The listing builds one solid part. Answer for the finished solid, in the listing's coordinates (mm). Face numbers are marked on the shaded views. A direction names the side the tool comes from. Give positions to 0.01 mm unless a question says otherwise; leave off trailing zeros. Order: outer loops, then holes, each group sorted by start corner. A loop starts at its lowest first (then second) coordinate and runs counter-clockwise, first axis right, second up. Notation, with made-up numbers: M -15,-14 L 29,-14 A24 ccw 29,-3 Z; hole C 70.25,64 d9. An arc over 180 degrees is marked long. Answer as a JSON object with one key per item and string values. Group by question number.
```python
from build123d import *

# Parameters (mm, degrees)
F0_W        = 63.5
F0_H        = 50.8
F1_DEPTH    = 3.175
F2_R        = 22.621875
F3_DEPTH    = 1.27
F5_DEPTH    = 25.4
F7_DEPTH    = 50.8
F8_T1_DEPTH = 50.8
F8_T3_DEPTH = 74.3464301965
F8_T5_DEPTH = 76.2
F9_R        = 5.08
F10_R       = 1.27


# Not quite as in the source:
# - a fillet or chamfer that OpenCascade refuses, or shapes differently, is made with other operations: its cross-section is extruded or revolved along the edge and cut away or added


with BuildPart() as f1:
    # F0 (on Right) → F1 (new body)
    with BuildSketch(Plane.YZ):
        Rectangle(F0_W, F0_H)
    extrude(amount=F1_DEPTH)

    # F2 (on face) → F3 (cut)
    with BuildSketch(Plane.YZ.offset(3.175)):
        with Locations((2.778125, 0)):
            Circle(F2_R)
    extrude(amount=-F3_DEPTH, mode=Mode.SUBTRACT)

    # F4 (on face) → F5 (cut)
    with BuildSketch(Plane.YZ.offset(1.905)):
        with BuildLine():
            ThreePointArc((14.3248105234, 15.875), (11.3272476722, 18.1751108739), (9.8813375306, 14.684375))
            Line((9.8813375306, 14.684375), (11.9435605234, 15.875))
            Line((11.9435605234, 15.875), (11.9435605234, 13.49375))
            ThreePointArc((11.9435605234, 13.49375), (13.6273585461, 14.1912019773), (14.3248105234, 15.875))
        make_face()
        with BuildLine():
            Line((-15.5527460468, 0), (-13.490523054, 1.190625))
            ThreePointArc((-13.490523054, 1.190625), (-17.9339960468, 0), (-13.490523054, -1.190625))
            Line((-13.490523054, -1.190625), (-15.5527460468, 0))
        make_face()
        with BuildLine():
            ThreePointArc((-13.490523054, -1.190625), (-13.2526351729, -0.6163128512), (-13.1714960468, 0))
            Line((-13.1714960468, 0), (-15.5527460468, 0))
            Line((-15.5527460468, 0), (-13.490523054, -1.190625))
        make_face()
        with BuildLine():
            Line((-15.5527460468, 0), (-13.1714960468, 0))
            ThreePointArc((-13.1714960468, 0), (-13.2526351729, 0.6163128512), (-13.490523054, 1.190625))
            Line((-13.490523054, 1.190625), (-15.5527460468, 0))
        make_face()
        with BuildLine():
            ThreePointArc((10.7529355234, -13.8127770072), (10.2597625007, -14.1912019773), (9.8813375306, -14.684375))
            Line((9.8813375306, -14.684375), (11.9435605234, -15.875))
            Line((11.9435605234, -15.875), (10.7529355234, -13.8127770072))
        make_face()
        with BuildLine():
            Line((11.9435605234, 15.875), (10.7529355234, 13.8127770072))
            ThreePointArc((10.7529355234, 13.8127770072), (11.3272476722, 13.5748891261), (11.9435605234, 13.49375))
            Line((11.9435605234, 13.49375), (11.9435605234, 15.875))
        make_face()
        with BuildLine():
            Line((11.9435605234, 15.875), (9.8813375306, 14.684375))
            ThreePointArc((9.8813375306, 14.684375), (10.2597625007, 14.1912019773), (10.7529355234, 13.8127770072))
            Line((10.7529355234, 13.8127770072), (11.9435605234, 15.875))
        make_face()
        with BuildLine():
            Line((11.9435605234, -15.875), (9.8813375306, -14.684375))
            ThreePointArc((9.8813375306, -14.684375), (11.3272476722, -18.1751108739), (14.3248105234, -15.875))
            ThreePointArc((14.3248105234, -15.875), (13.6273585461, -14.1912019773), (11.9435605234, -13.49375))
            Line((11.9435605234, -13.49375), (11.9435605234, -15.875))
        make_face()
        with BuildLine():
            ThreePointArc((11.9435605234, -13.49375), (11.3272476722, -13.5748891261), (10.7529355234, -13.8127770072))
            Line((10.7529355234, -13.8127770072), (11.9435605234, -15.875))
            Line((11.9435605234, -15.875), (11.9435605234, -13.49375))
        make_face()
    extrude(amount=-F5_DEPTH, mode=Mode.SUBTRACT)

    # F6 (on face) → F7 (join, through all)
    with BuildSketch(Plane.XY.offset(25.4)):
        Polygon((-19.05, -31.75), (0, -31.75), (0, -28.575), (-15.875, -28.575), (-15.875, -22.225), (-19.05, -22.225), align=None)
    extrude(amount=-F7_DEPTH)

    # F8: fillet of radius 5.08 on 3 edges, made by hand

    # F8_s2 → F8_t1 (join)
    with BuildSketch(Plane.XY.offset(-25.4)):
        with BuildLine():
            ThreePointArc((-5.08, -28.575), (-1.4878975516, -27.0871024484), (0, -23.495))
            Line((0, -23.495), (0, -28.575))
            Line((0, -28.575), (-5.08, -28.575))
        make_face()
    extrude(amount=F8_T1_DEPTH)

    # F8_s4 → F8_t3 (cut)
    with BuildSketch(Plane.XY.offset(-37.1732150983)):
        with BuildLine():
            ThreePointArc((0, 31.75), (2.3071134838, 29.8805202921), (3.175, 27.0407139607))
            Line((3.175, 27.0407139607), (3.175, 31.75))
            Line((3.175, 31.75), (0, 31.75))
        make_face()
    extrude(amount=F8_T3_DEPTH, mode=Mode.SUBTRACT)

    # F8_s6 → F8_t5 (cut)
    with BuildSketch(Plane.XY.offset(-38.1)):
        with BuildLine():
            ThreePointArc((-19.05, -26.67), (-17.5621024484, -30.2621024484), (-13.97, -31.75))
            Line((-13.97, -31.75), (-19.05, -31.75))
            Line((-19.05, -31.75), (-19.05, -26.67))
        make_face()
    extrude(amount=F8_T5_DEPTH, mode=Mode.SUBTRACT)

    # F9
    f9_edges = [f1.edges().sort_by_distance(p)[0] for p in [
        (3.175, -31.75, 0),
    ]]
    fillet(f9_edges, radius=F9_R)

    # F10
    f10_edges = [f1.edges().sort_by_distance(p)[0] for p in [
        (0, 31.75, 0),
    ]]
    fillet(f10_edges, radius=F10_R)


solid = f1.part
```
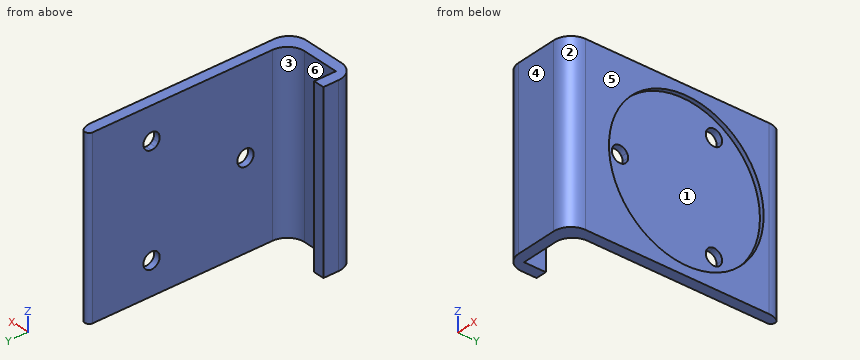
Item 1: Section D-D (x = -13.25) is taken. Determine the outline of the cut face in (y, z) (3 decimals).
Item 2: Flat-ended cylindrical pins translate along their axes: P1, Ø6, axis at y = 11.94, z = -15.88, coming from the -X side; P2, Ø1.5, axis at x = -15.5, z = 6, coming from the -Y side; P3, Ø2, axis at x = -2, z = -13.5, coming from the +Y side. Find the tip coordinate at first contact, or state that the pin passes through.
Item 3: Section A-A (y = -15) is taken. Determine the outline of the cut face in (x, z) (3 decimals).
Item 4: Consider probe 1 along X at (y, z) = (-7.5, 9.5) (3 decimals); probe 2 along Y at (x, z) = (-9.75, 15) (3 decimals); probe 3 along X at (y, z) = (24.5, -7) (3 decimals). Determine where each line is inside the solid, lowest interval first. Write a range as from..to.
Item 5: Section B-B (z = -17) is taken. Determine the outline of the cut face in (x, y) (3 decimals), and give its area (3 significant figures).
Item 6: Section C-C (y = 0) is taken. Determine the outline of the cut face in (x, z) (3 decimals), and give its area (3 significant figures).
Item 7: A tool of negligible diameter and unlimited length cuts with its end or side. For the marked faces 1, 2 and 3, from which of +Z, -Z, +X, -X, +Y, -Y can it reach the whole face along a straight path? Write none if from no direction.
Item 8: Determine the mould class of the marked faces 4, 5 and 6 for opening direction X: released by +X, released by -X, zero draft, split by the parting line, or undercut.
Values found:
{
 "1": {"outline": "M -31.75,-25.4 L -28.575,-25.4 L -28.575,25.4 L -31.75,25.4 Z"},
 "2": {"P1": "stops at x = 0", "P2": "stops at y = -31.69", "P3": "stops at y = -26.52"},
 "3": {"outline": "M 0,-25.4 L 3.175,-25.4 L 3.175,-13.989 L 1.905,-13.989 L 1.905,-2.316 L 0,-2.316 Z; M 0,2.316 L 1.905,2.316 L 1.905,13.989 L 3.175,13.989 L 3.175,25.4 L 0,25.4 Z"},
 "4": {"probe 1": "x = 0..1.905", "probe 2": "y = -31.75..-28.575", "probe 3": "x = 0..3.175"},
 "5": {"outline": "M -19.05,-26.67 A5.08 ccw -13.97,-31.75 L -1.905,-31.75 A5.08 ccw 3.175,-26.67 L 3.175,-12.147 L 1.905,-12.147 L 1.905,9.845 L 0,9.845 L 0,-23.495 A5.08 cw -5.08,-28.575 L -15.875,-28.575 L -15.875,-22.225 L -19.05,-22.225 Z; M 0,14.042 L 1.905,14.042 L 1.905,17.703 L 3.175,17.703 L 3.175,27.041 A5.08 ccw 2.328,29.849 A1.27 ccw 0,29.147 Z", "area": "225 mm^2"},
 "6": {"outline": "M 0,-25.4 L 3.175,-25.4 L 3.175,-22.451 L 1.905,-22.451 L 1.905,22.451 L 3.175,22.451 L 3.175,25.4 L 0,25.4 Z", "area": "104 mm^2"},
 "7": {"face 1": "+X", "face 2": "+Z, -Z, +X, -Y", "face 3": "+Z, -Z, +Y"},
 "8": {"face 4": "zero draft", "face 5": "released by +X", "face 6": "undercut"}
}
